Input: part model. Units: mm. Frame: model coordinates. Face numbers are marked on the shaded views. A direction names the side the tool comes from. Give positions to 0.01 mm unless a question says otherwise; leave off trailing zeros. Loops run counter-clockwise (first coordinate to the right, second up) from the corner with the lowest first, then second, coordinate; pieces in that order, holes last. Notation, with made-up numbers: M 41,83.25 L 77,83.25 A33 cw 77,120.25 Z; hole C 82,-29.75 d10. An arc over 180 degrees is marked long. One line per item, written item: value. Start each with the question number.
(1) Section B-B on x = -8.5. Output: boundary loops of the cut face in (y, z), plus the area to 3 significant figures.
(2) Ray query, line 1 along Y through (x, z) = (0, 10.8); line 2 along X through (y, z) = (-12, 6.5); line 3 along Z through (x, y) = (-7, 12). Return the intervals inside material, ascending. Write a range as from..to.
(3) Section A-A on y = -4. Output: boundary loops of the cut face in (x, z), plus the area to 3 significant figures.
(4) Pull-direction query (Y, two-part tool) for the marked faces 6, 7 and 8; classes: released by +Y, released by -Y, zero draft, split by the parting line, or undercut.
(5) Pin query (flat end, axial travel): P1, Ø1.6, axis at x = 16.5, z = 3.5, coming from the +Y side; P2, Ø0.9, axis at x = -16.5, z = 2, coming from the -Y side; P3, Ø5, axis at x = -9.5, y = 6.5, coming from the -Z side; P4, Ø5, axis at y = -13, z = 11, coming from the +X side. Return the tip coordinate at first contact, or that it passes through.
(6) Section C-C on y = 17.5. Output: boundary loops of the cut face in (x, z).
(7) Access query for the marked faces 1, 2, 3, 4 and 5. Directions: +Z, -Z, +X, -X, +Y, -Y. A direction counts if a zero-diameter tool reaches every point of the face in a straight line with its end or side. Return the directions, or none.
```python
from build123d import *

# Parameters (mm, degrees)
CONTOUR_R                                    = 19
BOSS_EXTRU_1_CONTOUR_DEPTH                   = 13
COQUE1_T                                     = -3
ENL_V_MAT_EXTRU_1_OUVERTUE_AIMANT_REACH      = 46.43
ENL_V_MAT_EXTRU_1_OUVERTUE_AIMANT_END_RADIUS = 16
ENL_V_MAT_EXTRU_2_OUVERTURE_CROU_REACH       = 31.85
OUVERTURE_CROU_R                             = 13.5
BOSS_EXTRU_2_AILETTES_REACH                  = 51.216
BOSS_EXTRU_2_AILETTES_END_RADIUS             = 19
AILETTES_W                                   = 1.5
AILETTES_H                                   = 13
R_P_TITION_CIRCULAIRE4_AILETTES_COUNT        = 6
CONG_1_AILETTES_R                            = 0.75


with BuildPart() as part:
    # Contour → Boss.-Extru.1_Contour (new body)
    with BuildSketch(Plane.XY):
        with Locations(Location((0, 0, 0), (0, 0, 180))):
            Circle(CONTOUR_R)
    extrude(amount=BOSS_EXTRU_1_CONTOUR_DEPTH)

    # Coque1
    coque1_openings = [part.faces().sort_by_distance(p)[0] for p in [
        (0, 0, 0),
    ]]
    offset(amount=COQUE1_T, openings=coque1_openings, kind=Kind.INTERSECTION)

    # Enlèv. mat.-Extru.1_Ouvertue_aimant: up to this cylinder (the profile starts outside it)
    enl_v_mat_extru_1_ouvertue_aimant_end = Plane(origin=(0, 0, 4.533251), z_dir=(0, 0, -1)) * Cylinder(ENL_V_MAT_EXTRU_1_OUVERTUE_AIMANT_END_RADIUS, 125.86, mode=Mode.PRIVATE)
    # Ouvertue_aimant → Enlèv. mat.-Extru.1_Ouvertue_aimant (cut, up to the surface)
    with BuildSketch(Plane(origin=(19, 0, 0), x_dir=(0, 0, -1), z_dir=(1, 0, 0)), mode=Mode.PRIVATE) as enl_v_mat_extru_1_ouvertue_aimant_sk1:
        with BuildLine():
            Line((0, 5), (-5, 5))
            ThreePointArc((-5, 5), (-10, 0), (-5, -5))
            Line((-5, -5), (0, -5))
            Line((0, -5), (0, 5))
        make_face()
    enl_v_mat_extru_1_ouvertue_aimant_tool1 = extrude(enl_v_mat_extru_1_ouvertue_aimant_sk1.sketch, amount=-ENL_V_MAT_EXTRU_1_OUVERTUE_AIMANT_REACH, mode=Mode.PRIVATE) - enl_v_mat_extru_1_ouvertue_aimant_end
    enl_v_mat_extru_1_ouvertue_aimant = enl_v_mat_extru_1_ouvertue_aimant_tool1.solids().sort_by_distance((19, 0, 4.533251))[0]
    add(enl_v_mat_extru_1_ouvertue_aimant, mode=Mode.SUBTRACT)

    # Symétrie1_Ouvertue_aimant: Enlèv. mat.-Extru.1_Ouvertue_aimant across plane
    add(enl_v_mat_extru_1_ouvertue_aimant.mirror(Plane(origin=(0, 0, 0), x_dir=(0, 0, 1), z_dir=(1, 0, 0))), mode=Mode.SUBTRACT)

    # Ouverture_Écrou → Enlèv. mat.-Extru.2_Ouverture_Écrou (cut, up to next)
    with BuildSketch(Plane.XY.offset(13), mode=Mode.PRIVATE) as enl_v_mat_extru_2_ouverture_crou_sk1:
        Circle(OUVERTURE_CROU_R)
    enl_v_mat_extru_2_ouverture_crou_tool1 = extrude(enl_v_mat_extru_2_ouverture_crou_sk1.sketch, amount=-ENL_V_MAT_EXTRU_2_OUVERTURE_CROU_REACH, mode=Mode.PRIVATE) & part.part
    add(enl_v_mat_extru_2_ouverture_crou_tool1.solids().sort_by_distance((0, 0, 13))[0], mode=Mode.SUBTRACT)

    # Boss.-Extru.2_Ailettes: up to this cylinder (the profile starts outside it)
    boss_extru_2_ailettes_end = Plane(origin=(0, 0, 6.5), z_dir=(0, 0, -1)) * Cylinder(BOSS_EXTRU_2_AILETTES_END_RADIUS, 141.432, mode=Mode.PRIVATE)
    # Ailettes → Boss.-Extru.2_Ailettes (add, up to the surface)
    with BuildSketch(Plane(origin=(0, 24.5, 0), x_dir=(1, 0, 0), z_dir=(0, 1, 0)), mode=Mode.PRIVATE) as boss_extru_2_ailettes_sk1:
        with Locations((0, -6.5)):
            Rectangle(AILETTES_W, AILETTES_H)
    boss_extru_2_ailettes_tool1 = extrude(boss_extru_2_ailettes_sk1.sketch, amount=-BOSS_EXTRU_2_AILETTES_REACH, mode=Mode.PRIVATE) - boss_extru_2_ailettes_end
    boss_extru_2_ailettes = boss_extru_2_ailettes_tool1.solids().sort_by_distance((0, 24.5, 6.5))[0]
    add(boss_extru_2_ailettes)

    # Répétition circulaire4_Ailettes: Boss.-Extru.2_Ailettes ×6 about axis
    r_p_tition_circulaire4_ailettes_axis = Axis((0, 0, 0), (0, 0, 1))
    for i in range(1, R_P_TITION_CIRCULAIRE4_AILETTES_COUNT):
        add(boss_extru_2_ailettes.rotate(r_p_tition_circulaire4_ailettes_axis, i * 360 / R_P_TITION_CIRCULAIRE4_AILETTES_COUNT))

    # Congé1_Ailettes
    cong_1_ailettes_edges = [part.edges().sort_by_distance(p)[0] for p in [
        (-20.842622393, -12.899519053, 6.5),
        (-21.217622393, -12.25, 13),
        (-21.592622393, -11.600480947, 6.5),
        (-21.217622393, -12.25, 0),
        (-21.592622393, 11.600480947, 6.5),
        (-21.217622393, 12.25, 13),
        (-20.842622393, 12.899519053, 6.5),
        (-21.217622393, 12.25, 0),
        (-0.75, 24.5, 6.5),
        (0, 24.5, 13),
        (0.75, 24.5, 6.5),
        (0, 24.5, 0),
        (20.842622393, 12.899519053, 6.5),
        (21.217622393, 12.25, 13),
        (21.592622393, 11.600480947, 6.5),
        (21.217622393, 12.25, 0),
        (21.592622393, -11.600480947, 6.5),
        (21.217622393, -12.25, 13),
        (20.842622393, -12.899519053, 6.5),
        (21.217622393, -12.25, 0),
        (0.75, -24.5, 6.5),
        (0, -24.5, 13),
        (-0.75, -24.5, 6.5),
        (0, -24.5, 0),
    ]]
    fillet(cong_1_ailettes_edges, radius=CONG_1_AILETTES_R - 0.0001)  # a hair under: the kernel refuses the full size


solid = part.part
```
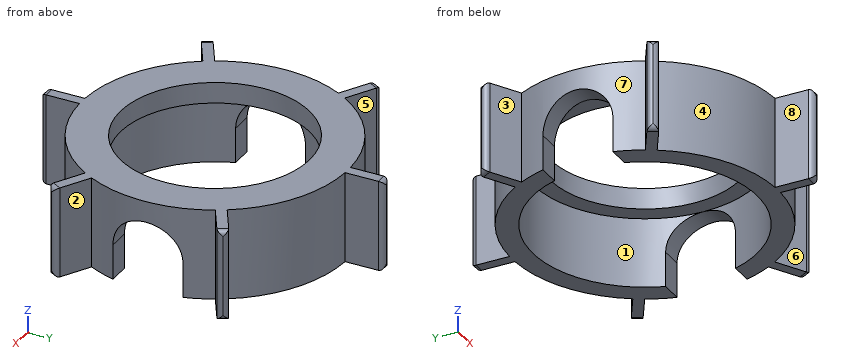
Output values:
1. outline: M -16.99,0 L -13.56,0 L -13.56,10 L -10.49,10 L -10.49,13 L -16.99,13 Z; M 10.49,10 L 13.56,10 L 13.56,0 L 16.99,0 L 16.99,13 L 10.49,13 Z
1. area: 108 mm²
2. line 1: y = -24.5..-13.5, 13.5..24.5
2. line 2: x = -21.31..-19.28, -14.73..-10.58, 10.58..14.73, 19.28..21.31
2. line 3: z = 10..13
3. outline: M -18.57,8 L -15.49,8 L -15.49,10 L -12.89,10 L -12.89,13 L -18.57,13 Z; M 12.89,10 L 15.49,10 L 15.49,8 L 18.57,8 L 18.57,13 L 12.89,13 Z
3. area: 46.4 mm²
4. face 6: released by -Y
4. face 7: undercut
4. face 8: zero draft
5. P1: stops at y = 10.85
5. P2: stops at y = -10.65
5. P3: stops at z = 10
5. P4: stops at x = 21.32
6. outline: M -7.4,0 L 7.4,0 L 7.4,13 L -7.4,13 Z
7. face 1: -Z
7. face 2: +Z, -Z, +X
7. face 3: +Z, -Z, -X
7. face 4: +Z, -Z, -Y
7. face 5: +Z, -Z, +Y
